```python
from build123d import *

# Parameters (mm, degrees)
BOSS_EXTRUDE1_DEPTH = 1.8
SKETCH3_W           = 12
SKETCH3_H           = 3.48629
CUT_EXTRUDE1_DEPTH  = 0.6
SKETCH4_R           = 2.9
BOSS_EXTRUDE2_DEPTH = 4.2
CUT_EXTRUDE2_REACH  = 22.557
SKETCH5_R           = 0.8


with BuildPart() as part:
    # Sketch2 → Boss-Extrude1 (new body)
    with BuildSketch(Plane(origin=(0, 0, 0), x_dir=(1, 0, 0), z_dir=(0, 1, 0))):
        with BuildLine():
            Line((0, 0), (0, 9.98629))
            ThreePointArc((0, 9.98629), (6, 15.98629), (12, 9.98629))
            Line((12, 9.98629), (12, 0))
            Line((12, 0), (0, 0))
        make_face()
    extrude(amount=BOSS_EXTRUDE1_DEPTH)

    # Sketch3 → Cut-Extrude1 (cut)
    with BuildSketch(Plane(origin=(0, 1.8, 0), x_dir=(1, 0, 0), z_dir=(0, 1, 0))):
        with Locations((6, 1.743145)):
            Rectangle(SKETCH3_W, SKETCH3_H)
    extrude(amount=-CUT_EXTRUDE1_DEPTH, mode=Mode.SUBTRACT)

    # Sketch4 → Boss-Extrude2 (add)
    with BuildSketch(Plane(origin=(0, 1.8, 0), x_dir=(1, 0, 0), z_dir=(0, 1, 0))):
        with Locations(Location((6, 9.98629, 0), (0, 0, 90))):
            Circle(SKETCH4_R)
    extrude(amount=BOSS_EXTRUDE2_DEPTH)

    # Sketch5 → Cut-Extrude2 (cut, up to next)
    with BuildSketch(Plane(origin=(0, 1.2, 0), x_dir=(1, 0, 0), z_dir=(0, 1, 0)), mode=Mode.PRIVATE) as cut_extrude2_sk1:
        with Locations(Location((3, 1.743145, 0), (0, 0, 270))):
            Circle(SKETCH5_R)
    cut_extrude2_tool1 = extrude(cut_extrude2_sk1.sketch, amount=-CUT_EXTRUDE2_REACH, mode=Mode.PRIVATE) & part.part
    # Sketch5 → Cut-Extrude2 (cut, up to next)
    with BuildSketch(Plane(origin=(0, 1.2, 0), x_dir=(1, 0, 0), z_dir=(0, 1, 0)), mode=Mode.PRIVATE) as cut_extrude2_sk2:
        with Locations(Location((9, 1.743145, 0), (0, 0, 270))):
            Circle(SKETCH5_R)
    cut_extrude2_tool2 = extrude(cut_extrude2_sk2.sketch, amount=-CUT_EXTRUDE2_REACH, mode=Mode.PRIVATE) & part.part
    add(cut_extrude2_tool1.solids().sort_by_distance((3, 1.2, -1.743145))[0], mode=Mode.SUBTRACT)
    add(cut_extrude2_tool2.solids().sort_by_distance((9, 1.2, -1.743145))[0], mode=Mode.SUBTRACT)


solid = part.part
```
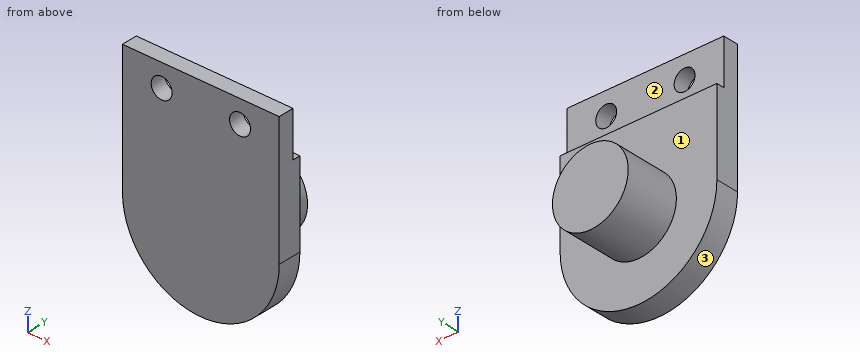
Work out the finished part from the listing and answer in its coordinate system (mm). Face numbers are marked on the shaded views. A direction names the side the tool comes from. Coordinates: 2 decimals unless noted, no trailing zeros. Loops run counter-clockwise (first coordinate to the right, second up) from the corner with the lowest first, then second, coordinate; pieces in that order, holes last. Notation, with made-up numbers: M 54.25,28 L 87.25,28 A21 cw 87.25,54 Z; hole C -15,55 d9. An arc over 180 degrees is marked long. Use CSV: the item, a comma, the result in double quotes. Start each with the question number.
(1) Consider line 1 (Y direction, x = 1.75, z = -7.5); line 2 (X direction, y = 1.5, z = -11.25); line 3 (Z direction, x = 5, y = 4.65). Determine where each line is inside the solid, lowest interval first.
(2) Given pin 1 Ø6 at (x, z) = (3.5, -12) entering from +Y; pin 2 Ø2 at (x, y) = (3, 2.5) entering from -Z; pin 3 Ø1 at (y, z) = (4, -8.5) entering from -X; pin 4 Ø2.5 at (x, z) = (9, -1.74) entering from +Y, each flat-ended and moving along its own axis, determine where each tip first touches the part or whether it passes through.
(3) Find section B-B, the plane y = 0.7. Give the vertices of the cut face in (x, z), then the cut area to 3 significant figures.
(4) For the marked faces 1, 2 and 3, determine the directions among +Z, -Z, +X, -X, +Y, -Y from which every point of the face is accessible in a straight line to the end or side of a thin tool.
(5) Find section A-A, the plane x = 6. Give the vertices of the cut face in (y, z).
(6) Find section D-D, the plane y = 3.65. Give the vertices of the cut face in (x, z), then the cut area to 3 significant figures.
(7) Find section C-C, the plane z = -5. Give the vertices of the cut face in (x, y).
Recorded:
1,line 1,"y = 0 to 1.8"
1,line 2,"x = 0.13 to 11.87"
1,line 3,"z = -12.71 to -7.26"
2,pin 1,"stops at y = 6"
2,pin 2,"stops at z = -15.53"
2,pin 3,"stops at x = 3.27"
2,pin 4,"stops at y = 1.2"
3,outline,"M 0,-9.99 A6 ccw 12,-9.99 L 12,0 L 0,0 Z; hole C 3,-1.74 d1.6; hole C 9,-1.74 d1.6"
3,area,"172 mm^2"
4,face 1,"+Y"
4,face 2,"+Z, +X, -X, +Y"
4,face 3,"-Z, +Y, -Y"
5,outline,"M 0,-15.99 L 1.8,-15.99 L 1.8,-12.89 L 6,-12.89 L 6,-7.09 L 1.8,-7.09 L 1.8,-3.49 L 1.2,-3.49 L 1.2,0 L 0,0 Z"
6,outline,"C 6,-9.99 d5.8"
6,area,"26.4 mm^2"
7,outline,"M 0,0 L 12,0 L 12,1.8 L 0,1.8 Z"
